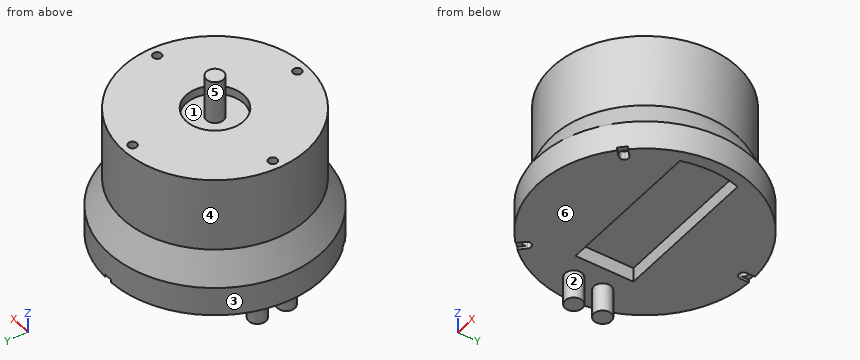
from build123d import *

# Parameters (mm, degrees)
SKETCH_1_R          = 32
EXTRUDE_1_DEPTH     = 25.5
SKETCH_3_R          = 37
EXTRUDE_3_DEPTH     = 10
SKETCH_4_R          = 1.5
CUT_EXTRUDE_1_DEPTH = 10
CUT_EXTRUDE_2_DEPTH = 5
SKETCH_7_R          = 3
EXTRUDE_4_DEPTH     = 10
CUT_EXTRUDE_START   = -1
CUT_EXTRUDE_3_DEPTH = 1
CUT_EXTRUDE_START_2 = -3
CUT_EXTRUDE_4_DEPTH = 3
SKETCH_9_R          = 10
SKETCH_9_R_2        = 3
CUT_EXTRUDE_5_DEPTH = 3
EXTRUDE_START       = 12
SKETCH_9_4_R        = 3
EXTRUDE_5_DEPTH     = 12


with BuildPart() as part:
    # Sketch 1 → Extrude 1 (new body)
    with BuildSketch(Plane.XY):
        Circle(SKETCH_1_R)
    extrude(amount=-EXTRUDE_1_DEPTH)



with BuildPart() as body_2:
    # Sketch 3 → Extrude 3 (new body)
    with BuildSketch(Plane(origin=(0, 0, -35.5), x_dir=(-1, 0, 0), z_dir=(0, 0, -1))):
        Circle(SKETCH_3_R)
    extrude(amount=EXTRUDE_3_DEPTH)


with BuildPart() as part_1:
    add(part.part)

    add(body_2.part)  # loft_1 joins it to this body
    # loft up to a face of the part (loft_1)
    loft([Face(Wire([part_1.edges().sort_by_distance((-21.90550739, -23.326996077, -25.5))[0]])), Face(Wire([part_1.edges().sort_by_distance((25.328242919, -26.971839215, -35.5))[0]]))])

    # Sketch 4 → Cut-Extrude 1 (cut)
    with BuildSketch(Plane.XY):
        with Locations((28.5, 0)):
            Circle(SKETCH_4_R)
        with Locations((0, -28.5)):
            Circle(SKETCH_4_R)
        with Locations((-28.5, 0)):
            Circle(SKETCH_4_R)
        with Locations((0, 28.5)):
            Circle(SKETCH_4_R)
    extrude(amount=-CUT_EXTRUDE_1_DEPTH, mode=Mode.SUBTRACT)

    # Sketch 5 → Cut-Extrude 2 (cut)
    with BuildSketch(Plane(origin=(0, 0, -45.5), x_dir=(-1, 0, 0), z_dir=(0, 0, -1))):
        with BuildLine():
            Line((0, -10), (0, 0))
            Line((0, 0), (0, 10))
            Line((0, 10), (-31.448370387, 10))
            ThreePointArc((-31.448370387, 10), (-33, 0), (-31.448370387, -10))
            Line((-31.448370387, -10), (0, -10))
        make_face()
        Polygon((20, -10), (0, -10), (0, 0), (0, 10), (20, 10), align=None)
    extrude(amount=-CUT_EXTRUDE_2_DEPTH, mode=Mode.SUBTRACT)

    # Sketch 7 → Extrude 4 (add)
    with BuildSketch(Plane(origin=(0, 0, -45.5), x_dir=(-1, 0, 0), z_dir=(0, 0, -1))):
        with Locations((28, 5)):
            Circle(SKETCH_7_R)
        with Locations((28, -5)):
            Circle(SKETCH_7_R)
    extrude(amount=EXTRUDE_4_DEPTH)

    # Sketch 8 → Cut-Extrude 3 (cut)
    with BuildSketch(Plane(origin=(0, 0, -45.5), x_dir=(-1, 0, 0), z_dir=(0, 0, -1)).offset(CUT_EXTRUDE_START)):
        with BuildLine():
            Line((-1.632304903, 36.963976798), (-1.499003176, 33.945323885))
            ThreePointArc((-1.499003176, 33.945323885), (-1.07981808, 35.041149804), (0, 35.5))
            Line((0, 35.5), (0, 37))
            ThreePointArc((0, 37), (-0.816351176, 36.990993103), (-1.632304903, 36.963976798))
        make_face()
        with BuildLine():
            ThreePointArc((0, 35.5), (1.060660172, 35.060660172), (1.5, 34))
            Line((1.5, 34), (1.5, 36.969582091))
            ThreePointArc((1.5, 36.969582091), (0.750154192, 36.992394741), (0, 37))
            Line((0, 37), (0, 35.5))
        make_face()
        with BuildLine():
            ThreePointArc((26.162950904, -26.162950904), (26.68801229, -25.627134057), (27.202102366, -25.080782023))
            Line((27.202102366, -25.080782023), (25.102290732, -22.980970389))
            ThreePointArc((25.102290732, -22.980970389), (25.427449859, -23.467605412), (25.54163056, -24.04163056))
            ThreePointArc((25.54163056, -24.04163056), (25.427449859, -24.615655709), (25.102290732, -25.102290732))
            Line((25.102290732, -25.102290732), (26.162950904, -26.162950904))
        make_face()
        with BuildLine():
            Line((22.980970389, -25.102290732), (25.080782023, -27.202102366))
            ThreePointArc((25.080782023, -27.202102366), (25.627134057, -26.68801229), (26.162950904, -26.162950904))
            Line((26.162950904, -26.162950904), (25.102290732, -25.102290732))
            ThreePointArc((25.102290732, -25.102290732), (24.04163056, -25.54163056), (22.980970389, -25.102290732))
        make_face()
        with BuildLine():
            ThreePointArc((-26.162950904, -26.162950904), (-25.627245299, -26.68790547), (-25.08100879, -27.201893281))
            Line((-25.08100879, -27.201893281), (-22.980970389, -25.102290732))
            ThreePointArc((-22.980970389, -25.102290732), (-24.04163056, -25.54163056), (-25.102290732, -25.102290732))
            Line((-25.102290732, -25.102290732), (-26.162950904, -26.162950904))
        make_face()
        with BuildLine():
            Line((-25.102290732, -22.980970389), (-27.290652839, -24.984400486))
            ThreePointArc((-27.290652839, -24.984400486), (-26.733297281, -25.579890861), (-26.162950904, -26.162950904))
            Line((-26.162950904, -26.162950904), (-25.102290732, -25.102290732))
            ThreePointArc((-25.102290732, -25.102290732), (-25.54163056, -24.04163056), (-25.102290732, -22.980970389))
        make_face()
    extrude(amount=CUT_EXTRUDE_3_DEPTH, mode=Mode.SUBTRACT)

    # Sketch 8_3 → Cut-Extrude 4 (cut)
    with BuildSketch(Plane(origin=(0, 0, -45.5), x_dir=(-1, 0, 0), z_dir=(0, 0, -1)).offset(CUT_EXTRUDE_START_2)):
        with BuildLine():
            ThreePointArc((-22.54163056, -24.04163056), (-22.655811262, -23.467605412), (-22.980970389, -22.980970389))
            Line((-22.980970389, -22.980970389), (-24.04163056, -24.04163056))
            Line((-24.04163056, -24.04163056), (-22.980970389, -25.102290732))
            ThreePointArc((-22.980970389, -25.102290732), (-22.655811262, -24.615655709), (-22.54163056, -24.04163056))
        make_face()
        with BuildLine():
            Line((-22.980970389, -25.102290732), (-24.04163056, -24.04163056))
            Line((-24.04163056, -24.04163056), (-25.102290732, -25.102290732))
            ThreePointArc((-25.102290732, -25.102290732), (-24.04163056, -25.54163056), (-22.980970389, -25.102290732))
        make_face()
        with BuildLine():
            Line((-24.04163056, -24.04163056), (-22.980970389, -22.980970389))
            ThreePointArc((-22.980970389, -22.980970389), (-24.04163056, -22.54163056), (-25.102290732, -22.980970389))
            Line((-25.102290732, -22.980970389), (-24.04163056, -24.04163056))
        make_face()
        with BuildLine():
            Line((-25.102290732, -25.102290732), (-24.04163056, -24.04163056))
            Line((-24.04163056, -24.04163056), (-25.102290732, -22.980970389))
            ThreePointArc((-25.102290732, -22.980970389), (-25.54163056, -24.04163056), (-25.102290732, -25.102290732))
        make_face()
        with BuildLine():
            ThreePointArc((25.102290732, -22.980970389), (24.04163056, -22.54163056), (22.980970389, -22.980970389))
            Line((22.980970389, -22.980970389), (24.04163056, -24.04163056))
            Line((24.04163056, -24.04163056), (25.102290732, -22.980970389))
        make_face()
        with BuildLine():
            Line((25.102290732, -22.980970389), (24.04163056, -24.04163056))
            Line((24.04163056, -24.04163056), (25.102290732, -25.102290732))
            ThreePointArc((25.102290732, -25.102290732), (25.427449859, -24.615655709), (25.54163056, -24.04163056))
            ThreePointArc((25.54163056, -24.04163056), (25.427449859, -23.467605412), (25.102290732, -22.980970389))
        make_face()
        with BuildLine():
            Line((24.04163056, -24.04163056), (22.980970389, -22.980970389))
            ThreePointArc((22.980970389, -22.980970389), (22.54163056, -24.04163056), (22.980970389, -25.102290732))
            Line((22.980970389, -25.102290732), (24.04163056, -24.04163056))
        make_face()
        with BuildLine():
            Line((25.102290732, -25.102290732), (24.04163056, -24.04163056))
            Line((24.04163056, -24.04163056), (22.980970389, -25.102290732))
            ThreePointArc((22.980970389, -25.102290732), (24.04163056, -25.54163056), (25.102290732, -25.102290732))
        make_face()
        with BuildLine():
            Line((0, 34), (0, 32.5))
            ThreePointArc((0, 32.5), (1.060660172, 32.939339828), (1.5, 34))
            Line((1.5, 34), (0, 34))
        make_face()
        with BuildLine():
            Line((0, 35.5), (0, 34))
            Line((0, 34), (1.5, 34))
            ThreePointArc((1.5, 34), (1.060660172, 35.060660172), (0, 35.5))
        make_face()
        with BuildLine():
            ThreePointArc((-1.499003176, 33.945323885), (-1.041149804, 32.92018192), (0, 32.5))
            Line((0, 32.5), (0, 34))
            Line((0, 34), (-1.499003176, 33.945323885))
        make_face()
        with BuildLine():
            Line((-1.499003176, 33.945323885), (0, 34))
            Line((0, 34), (0, 35.5))
            ThreePointArc((0, 35.5), (-1.07981808, 35.041149804), (-1.499003176, 33.945323885))
        make_face()
    extrude(amount=CUT_EXTRUDE_4_DEPTH, mode=Mode.SUBTRACT)

    # Sketch 9 → Cut-Extrude 5 (cut)
    with BuildSketch(Plane.XY):
        Circle(SKETCH_9_R)
        Circle(SKETCH_9_R_2, mode=Mode.SUBTRACT)
    extrude(amount=-CUT_EXTRUDE_5_DEPTH, mode=Mode.SUBTRACT)

    # Sketch 9_4 → Extrude 5 (add)
    with BuildSketch(Plane.XY.offset(EXTRUDE_START)):
        Circle(SKETCH_9_4_R)
    extrude(amount=-EXTRUDE_5_DEPTH)


solid = part_1.part
Here's how the part is built. I have some questions about the finished solid (model axes, mm). Face numbers are marked on the shaded views. A direction names the side the tool comes from. Coordinates: 2 decimals unless noted, no trailing zeros. Loops run counter-clockwise (first coordinate to the right, second up) from the corner with the lowest first, then second, coordinate; pieces in that order, holes last. Notation, with made-up numbers: (86.5, 41.25) -> (130.5, 41.25) arc R11 ccw to (130.5, 54.25) -> close; hole circle Ø6 at (4.5, -34). An arc over 180 degrees is marked (long way). Use one line per item in the form item = value. Start each with the question number.
(1) If we section it at B-B (z = -27.5): Please give me the cut outline in (x, y), then the cut area to 3 significant figures.
(2) We'd pull the mould along X, two halves only. Please class the marked faces 4, 5 and 6: pulls with the +X half, pulls with the -X half, needs draft (parallel to the pull), parting line crosses it, or undercut.
(3) Will these pins go through, and if not, where does the flat tip stop? pin 1 (1.3 mm diameter, centred on x = -25.5, y = -24.5, fed in from -Z); pin 2 (5 mm diameter, centred on y = 11, z = -40.5, fed in from +X); pin 3 (4.5 mm diameter, centred on x = 25, y = -25.5, fed in from -Z).
(4) If we section it at A-A (z = 4): Please give me the cut outline in (x, y), then the cut area to 3 significant figures.
(5) Please list where these lines run through material, in increasing order: line 1 along Y through (x, z) = (0, -7.75); line 2 along Z through (x, y) = (-5, -8); line 3 along Z through (x, y) = (24, 16).
(6) On a 3-axis mill with a long thin cutter (end or side, diameter ignored), from which of +Z, -Z, +X, -X, +Y, -Y can I reach the whole of each face in a straight line? I mean the marked faces 1, 2 and 3. Say none if no direction works.
Verdict:
q1.outline = circle Ø66 at (0, 0)
q1.area = 3,420 mm²
q2.face_4 = parting line crosses it
q2.face_5 = undercut
q2.face_6 = needs draft
q3.pin_1 = -44.5
q3.pin_2 = 36.01
q3.pin_3 = -45.5
q4.outline = circle Ø6 at (0, 0)
q4.area = 28.3 mm²
q5.line_1 = -32 to -30, -27 to 27, 30 to 32
q5.line_2 = -40.5 to -3
q5.line_3 = -45.5 to 0
q6.face_1 = +Z
q6.face_2 = -Z
q6.face_3 = +Z, -Z
